from build123d import *

# Parameters (mm, degrees)
SKETCH1_W                       = 40
SKETCH1_H                       = 20
BOSS_EXTRUDE1_DEPTH             = 7
SKETCH2_R                       = 0.5
CUT_EXTRUDE1_DEPTH              = 6.72
F_4_40_TAPPED_HOLE1_D           = 2.2606
F_4_40_TAPPED_HOLE1_CSINK_D     = 3.5306
F_4_40_TAPPED_HOLE1_CSINK_ANGLE = 90
LPATTERN1_COUNT                 = 2
LPATTERN1_PITCH                 = 30
SKETCH12_R                      = 5.55
SKETCH12_R_2                    = 3.97
CUT_EXTRUDE2_DEPTH              = 4.9
SKETCH13_W                      = 5
SKETCH13_H                      = 3.5
CUT_EXTRUDE3_DEPTH              = 0.5


with BuildPart() as part:
    # Sketch1 → Boss-Extrude1 (new body)
    with BuildSketch(Plane(origin=(0, 0, 0), x_dir=(1, 0, 0), z_dir=(0, 1, 0))):
        Rectangle(SKETCH1_W, SKETCH1_H)
    extrude(amount=BOSS_EXTRUDE1_DEPTH)

    # Sketch2 → Cut-Extrude1 (cut)
    with BuildSketch(Plane(origin=(0, 7, 0), x_dir=(1, 0, 0), z_dir=(0, 1, 0))):
        with Locations(Location((0, 0, 0), (0, 0, 270))):
            Circle(SKETCH2_R)
    extrude(amount=-CUT_EXTRUDE1_DEPTH, mode=Mode.SUBTRACT)

    # #4-40 Tapped Hole1 (through all)
    with Locations(Plane(origin=(-15, 0, 0), x_dir=(0, 0, -1), z_dir=(0, -1, 0))):
        with Locations((0, 0)):
            f_4_40_tapped_hole1 = CounterSinkHole(F_4_40_TAPPED_HOLE1_D / 2, F_4_40_TAPPED_HOLE1_CSINK_D / 2, counter_sink_angle=F_4_40_TAPPED_HOLE1_CSINK_ANGLE)

    # LPattern1: #4-40 Tapped Hole1 ×2
    with Locations(*[(i * LPATTERN1_PITCH, 0, 0) for i in range(1, LPATTERN1_COUNT)]):
        add(f_4_40_tapped_hole1, mode=Mode.SUBTRACT)

    # Sketch12 → Cut-Extrude2 (cut)
    with BuildSketch(Plane.XZ):
        with Locations(Location((0, 0, 0), (0, 0, 270))):
            Circle(SKETCH12_R)
        with Locations(Location((0, 0, 0), (0, 0, 270))):
            Circle(SKETCH12_R_2, mode=Mode.SUBTRACT)
    extrude(amount=-CUT_EXTRUDE2_DEPTH, mode=Mode.SUBTRACT)

    # Sketch13 → Cut-Extrude3 (cut)
    with BuildSketch(Plane.XZ):
        Rectangle(SKETCH13_W, SKETCH13_H)
    extrude(amount=-CUT_EXTRUDE3_DEPTH, mode=Mode.SUBTRACT)


solid = part.part
Geometry: final body of the model. Coordinates: model frame, mm. A direction names the side the tool comes from. Coordinates: 2 decimals unless noted, no trailing zeros. Loops run counter-clockwise (first coordinate to the right, second up) from the corner with the lowest first, then second, coordinate; pieces in that order, holes last. Notation, with made-up numbers: (-15.5, 72) - (12.5, 72) arc R20 ccw to (12.5, 96) - close; hole circle Ø6 at (48, 81.25). An arc over 180 degrees is marked (long way). One line per question, with ' | ' between items. Start each with the question number.
(1) Ray query, L1, parallel to X at y = 4, z = 0; L2, parallel to Z at x = -15, y = 2.75; L3, parallel to X at y = 3.75, z = -0.25. Return the intervals inside material, ascending. Write a range as from..to.
(2) Cut plane D-D on x = 15. Output: boundary loops of the cut face in (y, z) (3 decimals), and give its area (3 significant figures).
(3) Cut plane B-B on y = 4.25. Output: boundary loops of the cut face in (x, z).
(4) Cut plane A-A on x = 0. Output: boundary loops of the cut face in (y, z), and give its area (3 significant figures).
(5) Draft query along Z for faces 3 (the flat face through (0, 3, 10)), 4 (the cylindrical face through (-0.488, 3.796, -0.108)), 5 (the flat face through (0, 7, -2)). Return one class per face: +Z half, -Z half, draft (parallel to the pull), parting line (faces both ways), or undercut.
(6) Reachability of faces 1 (the flat face through (-1, 0.5, 0)), 2 (the flat face through (4, 0, -5)) from +Z, -Z, +X, -X, +Y, -Y: full face, straight path, thin tool, end or side. Return the list, or none.
(7) Cut plane C-C on z = 0. Count the separate pieces of the cut face and the enclosed holes in it, and give its area (3 significant figures).
(8) First-contact query: pin 1 (2.5 mm diameter, centred on x = 15, z = 0, fed in from -Y). Flat tip, straight axial feed; report the tip coordinate or a pass-through.
Here are the results:
1) L1: -20..-16.13, -13.87..-5.55, -3.97..-0.5, 0.5..3.97, 5.55..13.87, 16.13..20 | L2: -10..-1.13, 1.13..10 | L3: -20..-16.1, -13.9..-5.54, -3.96..-0.43, 0.43..3.96, 5.54..13.9, 16.1..20
2) outline: (0, -10) - (7, -10) - (7, -1.13) - (0.635, -1.13) - (0, -1.765) - close; (0, 1.765) - (0.635, 1.13) - (7, 1.13) - (7, 10) - (0, 10) - close | area: 124 mm²
3) outline: (-20, -10) - (20, -10) - (20, 10) - (-20, 10) - close; circle Ø7.94 at (0, 0); hole circle Ø2.26 at (-15, 0); hole circle Ø11.1 at (0, 0); hole circle Ø1 at (0, 0); hole circle Ø2.26 at (15, 0)
4) outline: (0, -10) - (7, -10) - (7, -0.5) - (0.5, -0.5) - (0.5, -1.75) - (0, -1.75) - (0, -3.97) - (4.9, -3.97) - (4.9, -5.55) - (0, -5.55) - close; (0, 1.75) - (0.5, 1.75) - (0.5, 0.5) - (7, 0.5) - (7, 10) - (0, 10) - (0, 5.55) - (4.9, 5.55) - (4.9, 3.97) - (0, 3.97) - close | area: 116 mm²
5) face 3: +Z half | face 4: undercut | face 5: draft
6) face 1: -Y | face 2: +Z, -Z, +X, -X, -Y
7) separate pieces: 4 | enclosed holes: 0 | area: 223 mm²
8) pin 1: y = 0.52
